The figure shows three views and two pictorial views of one solid part (mm, origin at its lowest corner). Answer the questions. Give positions to 0.01 mm unless a question says otherwise; leave off trailing zeros. Loops run counter-clockwise (first coordinate to the right, second up) from the corner with the lowest first, then second, coordinate; pieces in that order, holes last. Notation, with made-up numbers: (-13.75, 64) - (44.25, 64) arc R4 ccw to (44.25, 69) - close; hole circle Ø7 at (68, 7). An arc over 180 degrees is marked (long way). Use CSV: the item, a comma, the result in double quotes.
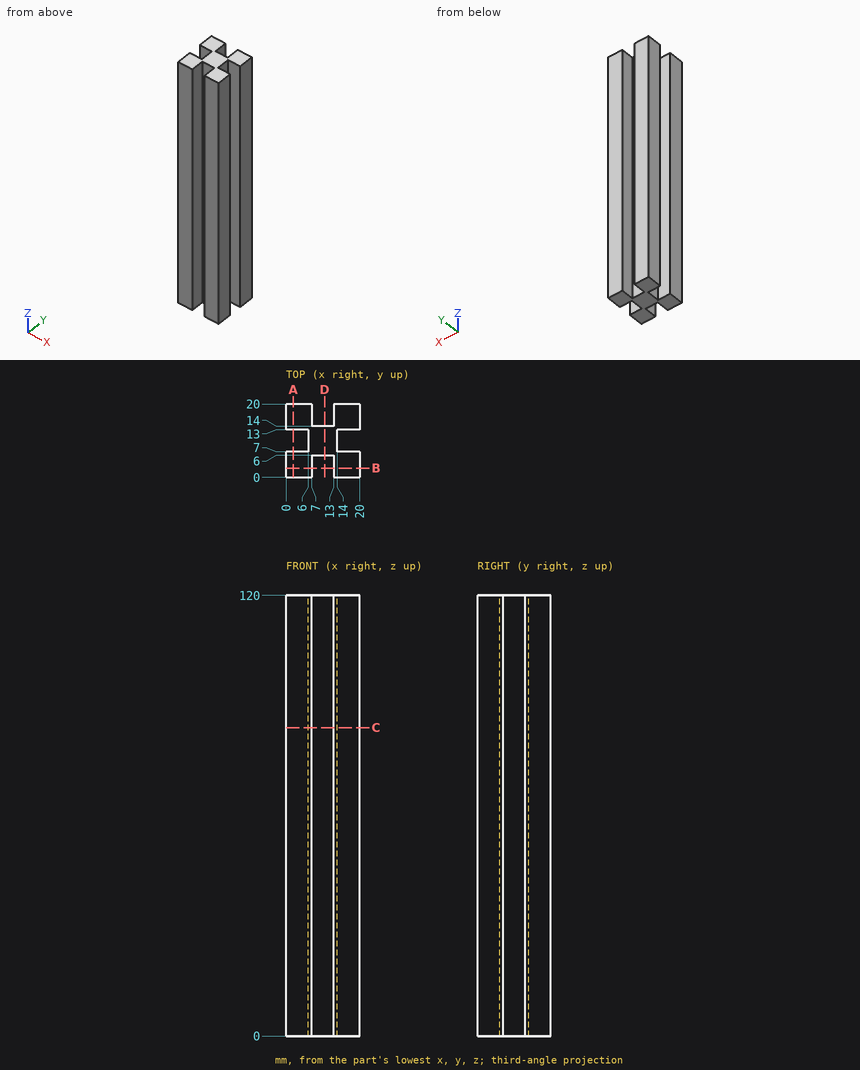
Item 1: A cutting plane is placed at D-D on x = 10.5. Determine the outline of the cut face in (y, z), and give its area (3 significant figures).
Determined:
outline,"(6, 0) - (14, 0) - (14, 120) - (6, 120) - close"
area,"960 mm²"
Item 2: Find the intervals of material crossed by line 1 (X direction, y = 5.5, z = 52.5); line 2 (X direction, y = 12.25, z = 20.5), in increasing order.
Determined:
line 1,"x = 0 to 7, 13 to 20"
line 2,"x = 6 to 14"
Item 3: A cutting plane is placed at A-A on x = 2. Determine the outline of the cut face in (y, z), and give its area (3 significant figures).
Determined:
outline,"(0, 0) - (7, 0) - (7, 120) - (0, 120) - close; (13, 0) - (20, 0) - (20, 120) - (13, 120) - close"
area,"1,680 mm²"
Item 4: A cutting plane is placed at C-C on z = 84. Determine the outline of the cut face in (x, y), and give its area (3 significant figures).
Determined:
outline,"(0, 0) - (7, 0) - (7, 6) - (13, 6) - (13, 0) - (20, 0) - (20, 7) - (14, 7) - (14, 13) - (20, 13) - (20, 20) - (13, 20) - (13, 14) - (7, 14) - (7, 20) - (0, 20) - (0, 13) - (6, 13) - (6, 7) - (0, 7) - close"
area,"256 mm²"
Item 5: Given P1, Ø3, axis at y = 9, z = 47.5, coming from the +X side, flat-ended and moving along its own axis, determine where the tip first touches the part or whether it passes through.
Determined:
P1,"stops at x = 14"
